Check sheet for the modelled part. Datum: model origin and axes. Units: mm. Face numbers are marked on the shaded views. A direction names the side the tool comes from. Give positions to 0.01 mm unless a question says otherwise; leave off trailing zeros. Loops run counter-clockwise (first coordinate to the right, second up) from the corner with the lowest first, then second, coordinate; pieces in that order, holes last. Notation, with made-up numbers: M -37.5,66.25 L -7.5,66.25 A12 ccw -7.5,74.25 Z; hole C 64.25,42 d6. An arc over 180 degrees is marked long. Write each question's results on one line, items separated by ' | '. Start each with the question number.
1. Material ranges on line 1 along Z through (x, y) = (19.5, 12); line 2 along Z through (x, y) = (16.5, 5.5); line 3 along Y through (x, z) = (16.25, 89.5), recorded low to high.
2. Tool access check on the marked faces 1, 2, 3, 4 and 5. Record the directions out of +Z, -Z, +X, -X, +Y, -Y that give a thin tool (end or side, any length) a straight path to the whole face; none if there is none.
3. Go/stop test with flat-tipped pins: pin 1 (3.5 mm diameter, centred on x = 18, y = -10, fed in from -Z); pin 2 (2 mm diameter, centred on x = 18, z = 52, fed in from -Y); pin 3 (4 mm diameter, centred on x = 7, y = 4.5, fed in from +Z). Record where each tip stops, or that it passes through.
4. Draft check along Z on the marked faces 6, 7 and 8. Enter one of: pulls with the +Z half, pulls with the -Z half, needs draft (parallel to the pull), parting line crosses it, or undercut.
5. Sectioned sample at D-D on z = 84. Record the cut outline in (x, y).
6. Sectioned sample at C-C on x = 19. Record the cut outline in (y, z).
7. Sectioned sample at A-A on y = 22.5. Record the cut outline in (x, z).
8. Sectioned sample at B-B on z = 46.5. Record the cut outline in (x, y), and give its area (3 significant figures).
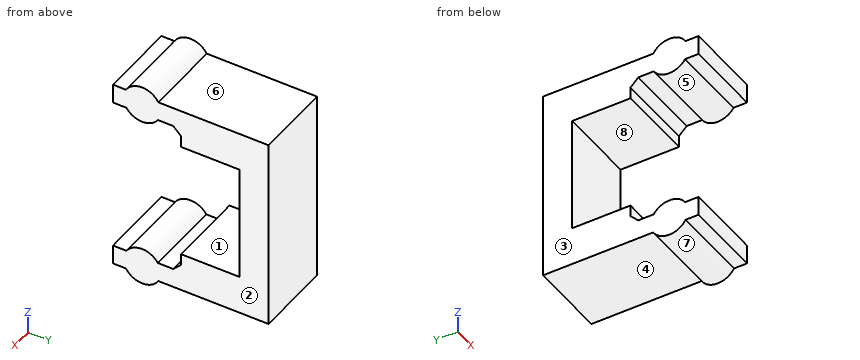
```python
from build123d import *

# Parameters (mm, degrees)
BOSS_EXTRUDE1_DEPTH = 25.4
SKETCH4_R           = 6.096
BOSS_EXTRUDE2_DEPTH = 25.4
CHAMFER1_SIZE       = 2.54


with BuildPart() as part:
    # Sketch3 → Boss-Extrude1 (new body)
    with BuildSketch(Plane(origin=(0, 0, 0), x_dir=(0, 0, -1), z_dir=(1, 0, 0))):
        Polygon((-101.845577666, -12.277652747), (-95.495577666, -12.277652747), (-95.495577666, 9.947347253), (-89.145577666, 9.947347253), (-89.145577666, 28.997347253), (-51.045577666, 28.997347253), (-51.045577666, 9.947347253), (-44.695577666, 9.947347253), (-44.695577666, -12.277652747), (-38.345577666, -12.277652747), (-38.345577666, 38.522347253), (-101.845577666, 38.522347253), align=None)
    extrude(amount=BOSS_EXTRUDE1_DEPTH)

    # Sketch4 → Boss-Extrude2 (add)
    with BuildSketch(Plane(origin=(25.4, 0, 0), x_dir=(0, 0, -1), z_dir=(1, 0, 0))):
        with Locations((-98.797577666, -2.752652747)):
            Circle(SKETCH4_R)
        with Locations((-41.393577666, -2.752652747)):
            Circle(SKETCH4_R)
    extrude(amount=-BOSS_EXTRUDE2_DEPTH)

    # Chamfer1
    chamfer1_edges = [part.edges().sort_by_distance(p)[0] for p in [
        (12.7, 9.947347253, 44.695577666),
        (12.7, 9.947347253, 95.495577666),
    ]]
    chamfer(chamfer1_edges, length=CHAMFER1_SIZE)


solid = part.part
```
Output values:
1) line 1: 38.35 to 51.05, 89.15 to 101.85 | line 2: 38.35 to 44.7, 95.5 to 101.85 | line 3: 9.95 to 38.52
2) face 1: +X, -X, -Y | face 2: +Z, -Z, +X, +Y, -Y | face 3: +Z, -Z, -X, +Y, -Y | face 4: -Z, +X, -X, +Y | face 5: +X, -X
3) pin 1: z = 38.35 | pin 2: y = 9.95 | pin 3: z = 101.89
4) face 6: pulls with the +Z half | face 7: pulls with the -Z half | face 8: undercut
5) outline: M 0,29 L 25.4,29 L 25.4,38.52 L 0,38.52 Z
6) outline: M -12.28,38.35 L -8.03,38.35 A6.1 ccw 2.53,38.35 L 38.52,38.35 L 38.52,101.85 L 2.53,101.85 A6.1 ccw -8.03,101.85 L -12.28,101.85 L -12.28,95.5 L -7.88,95.5 A6.1 ccw 2.37,95.5 L 7.41,95.5 L 9.95,92.96 L 9.95,89.15 L 29,89.15 L 29,51.05 L 9.95,51.05 L 9.95,47.24 L 7.41,44.7 L 2.37,44.7 A6.1 ccw -7.88,44.7 L -12.28,44.7 Z
7) outline: M 0,38.35 L 25.4,38.35 L 25.4,51.05 L 0,51.05 Z; M 0,89.15 L 25.4,89.15 L 25.4,101.85 L 0,101.85 Z
8) outline: M 0,-6.08 L 25.4,-6.08 L 25.4,0.58 L 0,0.58 Z; M 0,9.21 L 25.4,9.21 L 25.4,38.52 L 0,38.52 Z | area: 914 mm2
